```python
from build123d import *

# Parameters (mm, degrees)
SKETCH1_W            = 63
SKETCH1_H            = 50
BOSS_EXTRUDE1_DEPTH  = 28
CUT_EXTRUDE1_START   = -5
SKETCH2_W            = 60
SKETCH2_H            = 20
CUT_EXTRUDE1_DEPTH   = 62.748305375
CUT_EXTRUDE2_REACH   = 57.807
SKETCH3_W            = 40
SKETCH3_H            = 35
CUT_EXTRUDE3_REACH   = 57.807
SKETCH4_W            = 23
SKETCH4_H            = 25
SKETCH5_W            = 2.5
SKETCH5_H            = 25.5
BOSS_EXTRUDE2_DEPTH  = 35
SKETCH6_W            = 30
SKETCH6_H            = 15
CUT_EXTRUDE4_DEPTH   = 2.5
SKETCH7_W            = 2.5
SKETCH7_H            = 10.5
BOSS_EXTRUDE3_DEPTH  = 25
SKETCH8_W            = 5
SKETCH8_H            = 15
BOSS_EXTRUDE4_DEPTH  = 2.5
SKETCH9_W            = 10
SKETCH9_H            = 5.5
BOSS_EXTRUDE5_DEPTH  = 2.5
BOSS_EXTRUDE6_DEPTH  = 20
CUT_EXTRUDE6_START   = -5
CUT_EXTRUDE6_DEPTH   = 4
CUT_EXTRUDE8_START   = -5
CUT_EXTRUDE8_DEPTH   = 3
CUT_EXTRUDE9_DEPTH   = 64.548692085
SKETCH16_W           = 60.5
SKETCH16_H           = 5.5
CUT_EXTRUDE10_DEPTH  = 9
SKETCH17_W           = 10
SKETCH17_H           = 5.5
CUT_EXTRUDE11_DEPTH  = 18.5
SKETCH18_W           = 4.5
SKETCH18_H           = 5.5
BOSS_EXTRUDE7_DEPTH  = 34
SKETCH23_W           = 58
SKETCH23_H           = 45
CUT_EXTRUDE14_DEPTH  = 23
SKETCH24_W           = 2.5
SKETCH24_H           = 35
CUT_EXTRUDE15_DEPTH  = 3
BOSS_EXTRUDE9_START  = 56
SKETCH25_W           = 44
SKETCH25_H           = 2.5
BOSS_EXTRUDE9_DEPTH  = 3
SKETCH26_W           = 10
SKETCH26_H           = 20
BOSS_EXTRUDE10_DEPTH = 2.5
SKETCH27_W           = 44
SKETCH27_H           = 2.5
BOSS_EXTRUDE11_DEPTH = 6.5
SKETCH28_W           = 46.5
SKETCH28_H           = 2.5
BOSS_EXTRUDE12_DEPTH = 7
SKETCH29_W           = 46.5
SKETCH29_H           = 2.5
CUT_EXTRUDE16_DEPTH  = 4


with BuildPart() as part:
    # Sketch1 → Boss-Extrude1 (new body)
    with BuildSketch(Plane(origin=(0, 0, 0), x_dir=(1, 0, 0), z_dir=(0, 1, 0))):
        with Locations((2.724790291, -9.045064868)):
            Rectangle(SKETCH1_W, SKETCH1_H)
    extrude(amount=BOSS_EXTRUDE1_DEPTH)

    # Sketch2 → Cut-Extrude1 (cut, through all)
    with BuildSketch(Plane.XY.offset(34.045064868).offset(CUT_EXTRUDE1_START)):
        with Locations((1.724790291, 12.5)):
            Rectangle(SKETCH2_W, SKETCH2_H)
    extrude(amount=-CUT_EXTRUDE1_DEPTH, mode=Mode.SUBTRACT)

    # Cut-Extrude2: up to this face of the body (flat: up to its plane)
    cut_extrude2_end = Plane(part.part.faces().sort_by_distance((1.724790291, 2.5, 6.545064868))[0])
    # Sketch3 → Cut-Extrude2 (cut, up to the picked face)
    with BuildSketch(Plane(origin=(0, 28, 0), x_dir=(1, 0, 0), z_dir=(0, 1, 0)), mode=Mode.PRIVATE) as cut_extrude2_sk1:
        with Locations((-8.775209709, -1.545064868)):
            Rectangle(SKETCH3_W, SKETCH3_H)
    cut_extrude2_tool1 = split(extrude(cut_extrude2_sk1.sketch, amount=-CUT_EXTRUDE2_REACH, mode=Mode.PRIVATE), bisect_by=cut_extrude2_end, keep=Keep.BOTH, mode=Mode.PRIVATE)
    add(cut_extrude2_tool1.solids().sort_by(Axis((-8.77521, 28, 1.545065), (0, -1, 0)))[0], mode=Mode.SUBTRACT)

    # Cut-Extrude3: up to this face of the body (flat: up to its plane)
    cut_extrude3_end = Plane(part.part.faces().sort_by_distance((1.529988083, 2.5, 6.512866155))[0])
    # Sketch4 → Cut-Extrude3 (cut, up to the picked face)
    with BuildSketch(Plane(origin=(0, 28, 0), x_dir=(1, 0, 0), z_dir=(0, 1, 0)), mode=Mode.PRIVATE) as cut_extrude3_sk1:
        with Locations((22.724790291, -6.545064868)):
            Rectangle(SKETCH4_W, SKETCH4_H)
    cut_extrude3_tool1 = split(extrude(cut_extrude3_sk1.sketch, amount=-CUT_EXTRUDE3_REACH, mode=Mode.PRIVATE), bisect_by=cut_extrude3_end, keep=Keep.BOTH, mode=Mode.PRIVATE)
    add(cut_extrude3_tool1.solids().sort_by(Axis((22.72479, 28, 6.545065), (0, -1, 0)))[0], mode=Mode.SUBTRACT)

    # Sketch5 → Boss-Extrude2 (add)
    with BuildSketch(Plane(origin=(0, 0, 19.045064868), x_dir=(-1, 0, 0), z_dir=(0, 0, -1))):
        with Locations((27.525209709, 15.25)):
            Rectangle(SKETCH5_W, SKETCH5_H)
    extrude(amount=BOSS_EXTRUDE2_DEPTH)

    # Sketch6 → Cut-Extrude4 (cut)
    with BuildSketch(Plane(origin=(34.224790291, 0, 0), x_dir=(0, 0, -1), z_dir=(1, 0, 0))):
        with Locations((-19.045064868, 20.5)):
            Rectangle(SKETCH6_W, SKETCH6_H)
    extrude(amount=-CUT_EXTRUDE4_DEPTH, mode=Mode.SUBTRACT)

    # Sketch7 → Boss-Extrude3 (add)
    with BuildSketch(Plane(origin=(0, 0, 19.045064868), x_dir=(-1, 0, 0), z_dir=(0, 0, -1))):
        with Locations((-32.974790291, 7.75)):
            Rectangle(SKETCH7_W, SKETCH7_H)
    extrude(amount=BOSS_EXTRUDE3_DEPTH)

    # Sketch8 → Boss-Extrude4 (add)
    with BuildSketch(Plane(origin=(31.724790291, 0, 0), x_dir=(0, 0, -1), z_dir=(1, 0, 0))):
        with Locations((-31.545064868, 20.5)):
            Rectangle(SKETCH8_W, SKETCH8_H)
    extrude(amount=BOSS_EXTRUDE4_DEPTH)

    # Sketch9 → Boss-Extrude5 (add)
    with BuildSketch(Plane(origin=(31.724790291, 0, 0), x_dir=(0, 0, -1), z_dir=(1, 0, 0))):
        with Locations((-24.045064868, 25.25)):
            Rectangle(SKETCH9_W, SKETCH9_H)
    extrude(amount=BOSS_EXTRUDE5_DEPTH)

    # Sketch11 → Boss-Extrude6 (add)
    with BuildSketch(Plane(origin=(0, 0, 0), x_dir=(0, 0, -1), z_dir=(1, 0, 0))):
        with BuildLine():
            Line((0.954935132, 0), (-19.045064868, 0))
            Line((-19.045064868, 0), (-19.045064868, -15))
            ThreePointArc((-19.045064868, -15), (-9.045064868, -25), (0.954935132, -15))
            Line((0.954935132, -15), (0.954935132, 0))
        make_face()
    extrude(amount=BOSS_EXTRUDE6_DEPTH)

    # Sketch12 → Cut-Extrude6 (cut)
    with BuildSketch(Plane.ZY.offset(CUT_EXTRUDE6_START)):
        with BuildLine():
            Line((19.045064868, -15), (19.045064868, 0))
            Line((19.045064868, 0), (-0.954935132, 0))
            Line((-0.954935132, 0), (-0.954935132, -15))
            ThreePointArc((-0.954935132, -15), (9.045064868, -25), (19.045064868, -15))
        make_face()
    extrude(amount=-CUT_EXTRUDE6_DEPTH, mode=Mode.SUBTRACT)

    # Sketch14 → Cut-Extrude8 (cut)
    with BuildSketch(Plane.ZY.offset(-9).offset(CUT_EXTRUDE8_START)):
        with BuildLine():
            Line((19.045064868, -15), (19.045064868, 0))
            Line((19.045064868, 0), (-0.954935132, 0))
            Line((-0.954935132, 0), (-0.954935132, -15))
            ThreePointArc((-0.954935132, -15), (9.045064868, -25), (19.045064868, -15))
        make_face()
    extrude(amount=-CUT_EXTRUDE8_DEPTH, mode=Mode.SUBTRACT)

    # Sketch15 → Cut-Extrude9 (cut, through all)
    with BuildSketch(Plane.ZY.offset(-17)):
        with BuildLine():
            Line((19.045064868, -15), (19.045064868, 0))
            Line((19.045064868, 0), (-0.954935132, 0))
            Line((-0.954935132, 0), (-0.954935132, -15))
            ThreePointArc((-0.954935132, -15), (9.045064868, -25), (19.045064868, -15))
        make_face()
    extrude(amount=-CUT_EXTRUDE9_DEPTH, mode=Mode.SUBTRACT)

    # Sketch16 → Cut-Extrude10 (cut)
    with BuildSketch(Plane(origin=(0, 0, 19.045064868), x_dir=(-1, 0, 0), z_dir=(0, 0, -1))):
        with Locations((-3.974790291, 25.25)):
            Rectangle(SKETCH16_W, SKETCH16_H)
    extrude(amount=-CUT_EXTRUDE10_DEPTH, mode=Mode.SUBTRACT)

    # Sketch17 → Cut-Extrude11 (cut)
    with BuildSketch(Plane.ZY.offset(-11.224790291)):
        with Locations((-10.954935132, 25.25)):
            Rectangle(SKETCH17_W, SKETCH17_H)
    extrude(amount=-CUT_EXTRUDE11_DEPTH, mode=Mode.SUBTRACT)

    # Sketch18 → Boss-Extrude7 (add)
    with BuildSketch(Plane.XY.offset(-5.954935132)):
        with Locations((31.974790291, 25.25)):
            Rectangle(SKETCH18_W, SKETCH18_H)
    extrude(amount=BOSS_EXTRUDE7_DEPTH)

    # Sketch23 → Cut-Extrude14 (cut)
    with BuildSketch(Plane(origin=(0, 2.5, 0), x_dir=(1, 0, 0), z_dir=(0, 1, 0))):
        with Locations((2.724790291, -6.545064868)):
            Rectangle(SKETCH23_W, SKETCH23_H)
    extrude(amount=CUT_EXTRUDE14_DEPTH, mode=Mode.SUBTRACT)

    # Sketch24 → Cut-Extrude15 (cut)
    with BuildSketch(Plane.XZ.offset(-22.5)):
        with Locations((32.974790291, 11.545064868)):
            Rectangle(SKETCH24_W, SKETCH24_H)
    extrude(amount=-CUT_EXTRUDE15_DEPTH, mode=Mode.SUBTRACT)

    # Sketch25 → Boss-Extrude9 (add)
    with BuildSketch(Plane.ZY.offset(-29.724790291).offset(BOSS_EXTRUDE9_START)):
        with Locations((6.045064868, 26.75)):
            Rectangle(SKETCH25_W, SKETCH25_H)
    extrude(amount=-BOSS_EXTRUDE9_DEPTH)

    # Sketch26 → Boss-Extrude10 (add)
    with BuildSketch(Plane.ZY.offset(28.775209709)):
        with Locations((24.045064868, 12.5)):
            Rectangle(SKETCH26_W, SKETCH26_H)
    extrude(amount=-BOSS_EXTRUDE10_DEPTH)

    # Sketch27 → Boss-Extrude11 (add)
    with BuildSketch(Plane.ZY.offset(-29.724790291)):
        with Locations((6.045064868, 26.75)):
            Rectangle(SKETCH27_W, SKETCH27_H)
    extrude(amount=BOSS_EXTRUDE11_DEPTH)

    # Sketch28 → Boss-Extrude12 (add)
    with BuildSketch(Plane(origin=(0, 0, 28.045064868), x_dir=(-1, 0, 0), z_dir=(0, 0, -1))):
        with Locations((0.025209709, 26.75)):
            Rectangle(SKETCH28_W, SKETCH28_H)
    extrude(amount=BOSS_EXTRUDE12_DEPTH)

    # Sketch29 → Cut-Extrude16 (cut)
    with BuildSketch(Plane(origin=(0, 0, 21.045064868), x_dir=(-1, 0, 0), z_dir=(0, 0, -1))):
        with Locations((0.025209709, 26.75)):
            Rectangle(SKETCH29_W, SKETCH29_H)
    extrude(amount=-CUT_EXTRUDE16_DEPTH, mode=Mode.SUBTRACT)


solid = part.part
```
Design review of the part built by this model. Coordinates are the model's own, in mm. A direction names the side the tool comes from. Give positions to 0.01 mm unless a question says otherwise; leave off trailing zeros. Order: outer loops, then holes, each group sorted by start corner. A loop starts at its lowest first (then second) coordinate and runs counter-clockwise, first axis right, second up. Notation, with made-up numbers: (-13.5, 43.5) - (-4.5, 43.5) arc R18 cw to (-4.5, 55.5) - close; hole circle Ø10 at (67, 44.5). An arc over 180 degrees is marked (long way). Use a Markdown table: item, result. Add a question column.
(1) Add section D-D on z = 26.5. Give the boundary of the cut face in (x, y), then the cut area to 3 significant figures.
(2) Machinability: for faces 1 (the face through (14, -12, 9)), 2 (the face through (33, 13, 12)), 3 (the face through (31.725, 9, 2)), which of the approach directions +Z, -Z, +X, -X, +Y, -Y give a long, thin tool a straight path to every point of the face, cutting with its end or side? Answer none if there is none.
(3) Clearance check with flat-ended pins moving along their axes: P1, Ø1.5, axis at x = 2, y = -5.5, coming from the -Z side; P2, Ø6, axis at y = -15, z = 11.5, coming from the +X side; P3, Ø6, axis at y = -17.5, z = 6.5, coming from the -X side; P4, Ø15, axis at x = 7, z = 7.5, coming from the -Y side. State where each tip first meets the part, or that it passes through.
(4) Add section A-A on z = -2. Give the boundary of the cut face in (x, y), then the cut area to 4 significant figures.
(5) Mouldability with a two-part tool opening along X and no side actions: class faces 4 (the face through (2, -8, -0.955)), 5 (the face through (-23.275, 27, 4)), 6 (the face through (0, -12, 9)), 7 (the face through (2, 2.5, 6)) as +X half, -X half, draft (parallel to the pull), parting line (faces both ways), or undercut.
(6) Wall thickness on probe 1 along Y at (x, z) = (30.5, 1); probe 2 along X at (y, z) = (6.5, 1.5); probe 3 along X at (y, z) = (-3.5, 18): over which ranges is each line inside the solid? List them lowest first. Write a range as [from, to].
(7) Add section C-C on x = 15. Give the boundary of the cut face in (y, z).
(8) Add section B-B on y = -7.5. Give the boundary of the cut face in (x, z).
Report:
| question | item | result |
|---|---|---|
| 1 | outline | (-28.78, 0) - (34.22, 0) - (34.22, 13) - (31.72, 13) - (31.72, 2.5) - (-26.28, 2.5) - (-26.28, 25.5) - (34.22, 25.5) - (34.22, 28) - (-28.78, 28) - close |
| 1 | area | 399 mm² |
| 2 | face 1 | +Z, -Z, +X, -Y |
| 2 | face 2 | +X |
| 2 | face 3 | -Z |
| 3 | P1 | stops at z = -0.95 |
| 3 | P2 | stops at x = 14 |
| 3 | P3 | stops at x = 0 |
| 3 | P4 | stops at y = -25 |
| 4 | outline | (-28.78, 0) - (34.22, 0) - (34.22, 13) - (31.72, 13) - (31.72, 2.5) - (-26.28, 2.5) - (-26.28, 25.5) - (-23.28, 25.5) - (-23.28, 28) - (-28.78, 28) - close; (23.22, 25.5) - (34.22, 25.5) - (34.22, 28) - (23.22, 28) - close |
| 4 | area | 282.5 mm² |
| 5 | face 4 | draft |
| 5 | face 5 | undercut |
| 5 | face 6 | -X half |
| 5 | face 7 | undercut |
| 6 | probe 1 | y = [0, 2.5], [25.5, 28] |
| 6 | probe 2 | x = [-28.78, -26.28], [31.72, 34.22] |
| 6 | probe 3 | x = [0, 5], [9, 14] |
| 7 | outline | (0, -15.95) - (2.5, -15.95) - (2.5, 29.05) - (25.5, 29.05) - (25.5, 25.05) - (28, 25.05) - (28, 34.05) - (0, 34.05) - close |
| 8 | outline | (0, -0.95) - (5, -0.95) - (5, 19.05) - (0, 19.05) - close; (9, -0.95) - (14, -0.95) - (14, 19.05) - (9, 19.05) - close |
